Check sheet for the drawn part. Datum: minimum x, y, z corner. Units: mm. Give positions to 0.01 mm unless a question says otherwise; leave off trailing zeros. Loops run counter-clockwise (first coordinate to the right, second up) from the corner with the lowest first, then second, coordinate; pieces in that order, holes last.
1. Cross-section at A-A, the plane z = 89.5. Record the cut outline in (x, y), plus the area to 3 significant figures.
2. Cross-section at B-B, the plane z = 121. Record the cut outline in (x, y).
3. Material ranges on L1, parallel to Y at x = 3, z = 58, recorded low to high.
4. Go/stop test with flat-tipped pins: pin 1 Ø5 at (x, y) = (10, 8.5) entering from +Z; pin 2 Ø1.9 at (x, y) = (9, 6) entering from -Z; pin 3 Ø2 at (x, z) = (16, 131) entering from -Y. Record where each tip stops, or that it passes through.
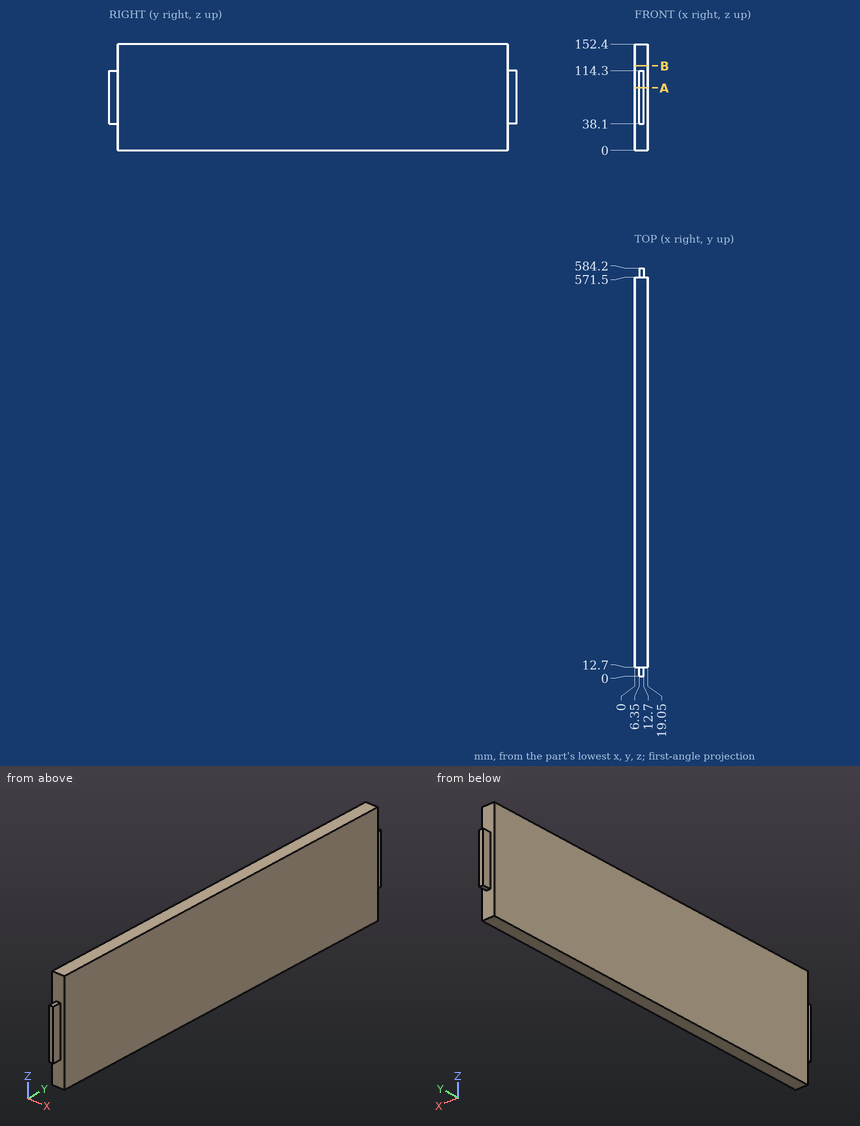
Result:
1. outline: (0, 12.7) - (6.35, 12.7) - (6.35, 0) - (12.7, 0) - (12.7, 12.7) - (19.05, 12.7) - (19.05, 571.5) - (12.7, 571.5) - (12.7, 584.2) - (6.35, 584.2) - (6.35, 571.5) - (0, 571.5) - close
1. area: 10,800 mm2
2. outline: (0, 12.7) - (19.05, 12.7) - (19.05, 571.5) - (0, 571.5) - close
3. L1: y = 12.7 to 571.5
4. pin 1: stops at z = 114.3
4. pin 2: stops at z = 38.1
4. pin 3: stops at y = 12.7
